Could you check a few things on this drawing? It's one solid part, dimensions in mm from its lowest x, y, z. A direction names the side the tool comes from. Coordinates: 2 decimals unless noted, no trailing zeros. Loops run counter-clockwise (first coordinate to the right, second up) from the corner with the lowest first, then second, coordinate; pieces in that order, holes last. Notation, with made-up numbers: (4.25, 61.25) -> (34.25, 61.25) arc R11 cw to (34.25, 81.25) -> close; hole circle Ø1 at (52.5, 17.25). An arc over 180 degrees is marked (long way). One line per question, with ' | ' between items. Start each with the question number.
(1) If we mould it in two halves opening along X, with no side actions, what happens to the marked faces 4, 5 and 6? For each: pulls with the +X half, pulls with the -X half, needs draft (parallel to the pull), parting line crosses it, or undercut.
(2) If I drill on line 1 along X through (y, z) = (36, 1.5); line 2 along X through (y, z) = (68, 2.25) (1 decimal); line 3 along X through (y, z) = (63.5, 1) (1 decimal), over which ranges is the centre line in solid material (lowest first)?
(3) Which directions (+Z, -Z, +X, -X, +Y, -Y) give clear straight access to the entire face, cutting with the end or side of a thin tool? Please do the marked faces 1, 2 and 3.
(4) I'm going to push flat-ended pins straight in: pin 1 Ø1.5 at (x, z) = (36.5, 3) entering from -Y; pin 2 Ø10 at (x, y) = (36.93, 67.39) entering from -Z; pin 3 Ø1.2 at (y, z) = (99, 3.5) entering from +X. Where does each tip first touch, or does it pass through?
(5) Suppose I cut it at D-D (y = 16). Please give me the cut outline in (x, z).
(6) Suppose I cut it at B-B (y = 66). Please give me the cut outline in (x, z), plus the area to 3 significant figures.
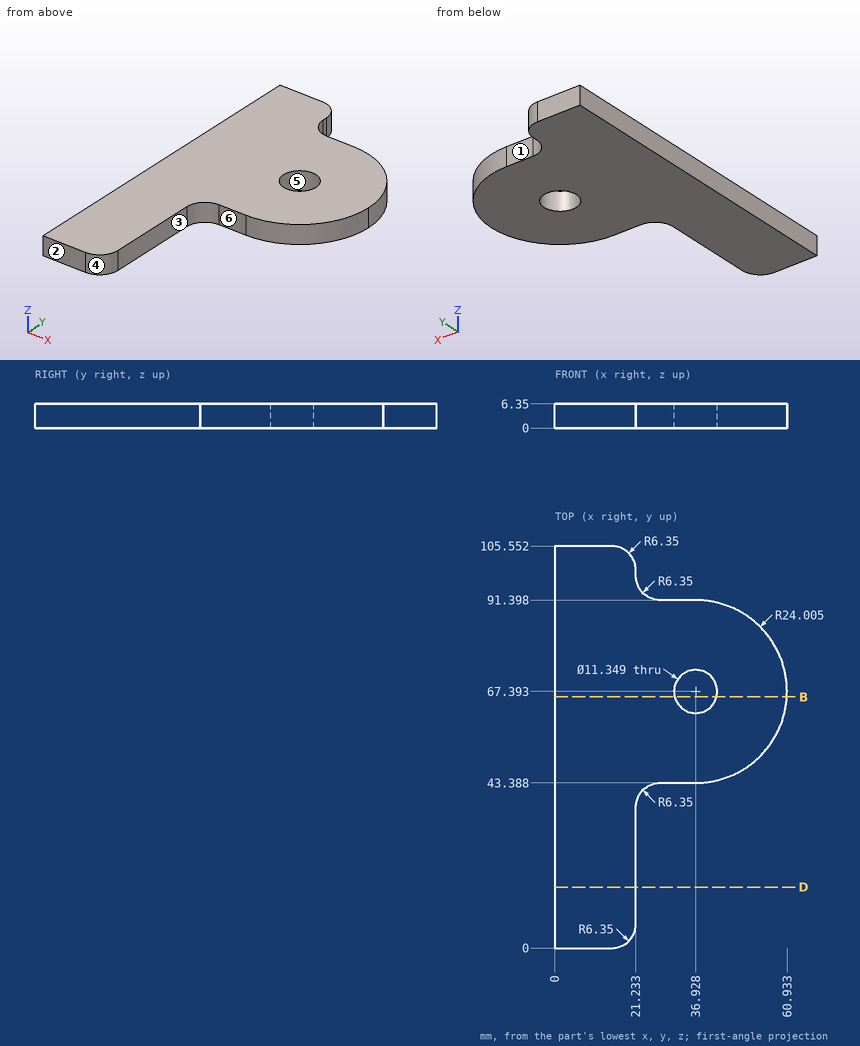
Checks:
1) face 4: pulls with the +X half | face 5: undercut | face 6: needs draft
2) line 1: x = 0 to 21.23 | line 2: x = 0 to 31.3, 42.6 to 60.9 | line 3: x = 0 to 32.8, 41.1 to 60.6
3) face 1: +Z, -Z, +X, +Y | face 2: +Z, -Z, +X, -X, -Y | face 3: +Z, -Z, +X, -Y
4) pin 1: stops at y = 43.39 | pin 2: passes through | pin 3: stops at x = 21.23
5) outline: (0, 0) -> (21.23, 0) -> (21.23, 6.35) -> (0, 6.35) -> close
6) outline: (0, 0) -> (31.43, 0) -> (31.43, 6.35) -> (0, 6.35) -> close; (42.43, 0) -> (60.89, 0) -> (60.89, 6.35) -> (42.43, 6.35) -> close | area: 317 mm^2
